Could you check a few things on this model? Use its own coordinates, in mm. Round coordinates to 2 decimals unless told otherwise and drop trailing zeros. Order: outer loops, then holes, each group sorted by start corner. A loop starts at its lowest first (then second) coordinate and runs counter-clockwise, first axis right, second up. Notation, with made-up numbers: (25.5, -27) -> (64.5, -27) arc R15 ccw to (64.5, -12) -> close; hole circle Ø3 at (9, -33.75). An arc over 180 degrees is marked (long way). One line per question, with ' | ' between items.
```python
from build123d import *

# Parameters (mm, degrees)
SKETCH1_R           = 6.35
EXTRUDE1_DEPTH      = 76.2
CHAMFER1_SIZE       = 0.9525
SKETCH3_W           = 3.175
SKETCH3_H           = 1.5875
EXTRUDE2_DEPTH      = 77.727341932
EXTRUDE2_DEPTH_BACK = 77.727341932
CHAMFER2_SIZE       = 1.373522526


with BuildPart() as part:
    # Sketch1 → Extrude1 (new, symmetric)
    with BuildSketch(Plane.XY):
        with Locations(Location((0, 0, 0), (0, 0, 180))):
            Circle(SKETCH1_R)
    extrude(amount=EXTRUDE1_DEPTH, both=True)

    # Chamfer1
    chamfer1_edges = [part.edges().sort_by_distance(p)[0] for p in [
        (6.35, 0, -76.2),
        (6.35, 0, 76.2),
    ]]
    chamfer(chamfer1_edges, length=CHAMFER1_SIZE)

    # Sketch3 → Extrude2 (cut, two sides)
    with BuildSketch(Plane.XY) as extrude2_sk:
        with Locations((0, 5.55625)):
            Rectangle(SKETCH3_W, SKETCH3_H)
    extrude(amount=EXTRUDE2_DEPTH, mode=Mode.SUBTRACT)
    extrude(extrude2_sk.sketch, amount=-EXTRUDE2_DEPTH_BACK, mode=Mode.SUBTRACT)

    # SurfaceCut1
    split(bisect_by=Plane.XY.offset(38.1), keep=Keep.BOTTOM)

    # Chamfer2
    chamfer2_edges = [part.edges().sort_by_distance(p)[0] for p in [
        (0, -6.35, 38.1),
    ]]
    chamfer(chamfer2_edges, length=CHAMFER2_SIZE)


solid = part.part
```
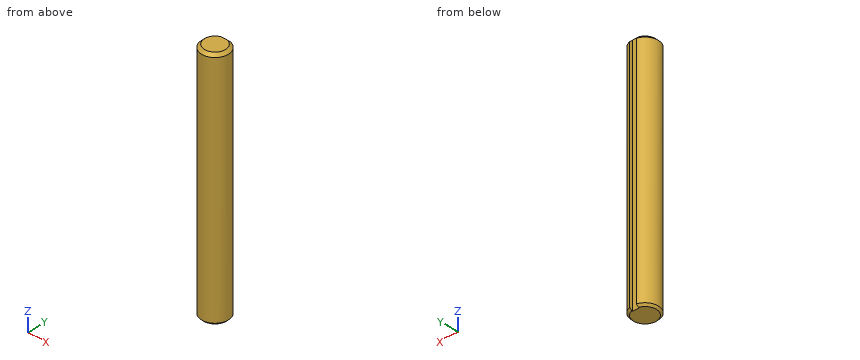
1. I want a section at A-A on x = 0. List the corners of the cut face in (y, z) for me, and give its area (3 significant figures).
From the geometry:
outline: (-6.35, -75.25) -> (-5.4, -76.2) -> (4.76, -76.2) -> (4.76, 38.1) -> (-4.98, 38.1) -> (-6.35, 36.73) -> close | area: 1,270 mm²
2. I'm going to push flat-ended pins straight in: pin 1 (1.1 mm diameter, centred on y = 5.5, z = -22.5, fed in from +X); pin 2 (1 mm diameter, centred on y = -4, z = -45.5, fed in from +X); pin 3 (5 mm diameter, centred on x = 3.5, z = 7.5, fed in from -Y). Where does each tip first touch, or does it pass through?
From the geometry:
pin 1: stops at x = 3.98 | pin 2: stops at x = 5.3 | pin 3: stops at y = -6.27
3. I need wall thicknesses on probe 1 along X at (y, z) = (5.75, 21); probe 2 along X at (y, z) = (-0.5, -63); probe 3 along Y at (x, z) = (-3.75, -69). Which ranges of each line are inside material? Lowest first, please.
From the geometry:
probe 1: x = -2.69 to -1.59, 1.59 to 2.69 | probe 2: x = -6.33 to 6.33 | probe 3: y = -5.12 to 5.12
4. I want a section at B-B on z = -3. List the corners of the cut face in (x, y) for me, and give its area (3 significant figures).
From the geometry:
outline: (-1.59, 4.76) -> (-1.59, 6.15) arc R6.35 ccw (long way) to (1.59, 6.15) -> (1.59, 4.76) -> close | area: 122 mm²
